from build123d import *

# Parameters (mm, degrees)
BOSS_EXTRUDE2_DEPTH           = 50
SKETCH2_R                     = 4.1
CUT_EXTRUDE1_DEPTH            = 50
SKETCH3_W                     = 12
SKETCH3_H                     = 24
CUT_EXTRUDE2_DEPTH            = 50
SKETCH4_R                     = 1.6
CUT_EXTRUDE3_DEPTH            = 50
CUT_EXTRUDE4_DEPTH            = 35
SKETCH6_R                     = 7.6
CUT_EXTRUDE5_DEPTH            = 35
CUT_EXTRUDE6_DEPTH            = 5.5
SKETCH8_R                     = 1.55
CUT_EXTRUDE7_DEPTH            = 116.876011322
CUT_EXTRUDE8_DEPTH            = 10
SKETCH10_R                    = 11
CUT_EXTRUDE9_DEPTH            = 29
SKETCH11_R                    = 1.05
SKETCH11_R_2                  = 4.75
CUT_EXTRUDE10_DEPTH           = 116.876011322
CUT_EXTRUDE11_DEPTH           = 2.5
FILLET1_R                     = 8
M3_TAPPED_HOLE3_D             = 2.5
M3_TAPPED_HOLE3_DEPTH         = 8.5
M3_TAPPED_HOLE3_CSINK_D       = 3.05
M3_TAPPED_HOLE3_CSINK_ANGLE   = 90
M3_TAPPED_HOLE3_TIP           = 0.751075774
M3_TAPPED_HOLE4_D             = 2.5
M3_TAPPED_HOLE4_DEPTH         = 7
M3_TAPPED_HOLE4_CSINK_D       = 3.05
M3_TAPPED_HOLE4_CSINK_ANGLE   = 90
M3_TAPPED_HOLE4_TIP           = 0.751075774
SKETCH15_R                    = 3.2
CUT_EXTRUDE12_DEPTH           = 1.5
CUT_EXTRUDE12_DRAFT           = -45
CUT_EXTRUDE12_PROFILE_2_DEPTH = 1.5
CUT_EXTRUDE12_PROFILE_2_DRAFT = -45
M3_TAPPED_HOLE5_D             = 2.5
M3_TAPPED_HOLE5_DEPTH         = 7
M3_TAPPED_HOLE5_CSINK_D       = 3.05
M3_TAPPED_HOLE5_CSINK_ANGLE   = 90
M3_TAPPED_HOLE5_TIP           = 0.751075774
SKETCH17_R                    = 3.2
CUT_EXTRUDE13_DEPTH           = 1.5
CUT_EXTRUDE13_DRAFT           = -45
CUT_EXTRUDE13_PROFILE_2_DEPTH = 1.5
CUT_EXTRUDE13_PROFILE_2_DRAFT = -45


with BuildPart() as part:
    # Sketch1 → Boss-Extrude2 (new body)
    with BuildSketch(Plane(origin=(0, 0, 0), x_dir=(0, 0, -1), z_dir=(1, 0, 0))):
        Polygon((0, 30), (0, 0), (-98.5, 0), (-98.5, 35), (5, 35), (5, 30), align=None)
    extrude(amount=BOSS_EXTRUDE2_DEPTH)

    # Sketch2 → Cut-Extrude1 (cut)
    with BuildSketch(Plane(origin=(50, 0, 0), x_dir=(0, 0, -1), z_dir=(1, 0, 0))):
        with Locations((-88.5, 26)):
            Circle(SKETCH2_R)
        with Locations((-8.5, 26)):
            Circle(SKETCH2_R)
    extrude(amount=-CUT_EXTRUDE1_DEPTH, mode=Mode.SUBTRACT)

    # Sketch3 → Cut-Extrude2 (cut)
    with BuildSketch(Plane(origin=(50, 0, 0), x_dir=(0, 0, -1), z_dir=(1, 0, 0))):
        with Locations((-24, 15)):
            Rectangle(SKETCH3_W, SKETCH3_H)
    extrude(amount=-CUT_EXTRUDE2_DEPTH, mode=Mode.SUBTRACT)

    # Sketch4 → Cut-Extrude3 (cut)
    with BuildSketch(Plane(origin=(50, 0, 0), x_dir=(0, 0, -1), z_dir=(1, 0, 0))):
        with Locations((-88.5, 16)):
            Circle(SKETCH4_R)
        with Locations((-68.5, 30)):
            Circle(SKETCH4_R)
        with Locations((-68.5, 5)):
            Circle(SKETCH4_R)
        with Locations((-8.5, 16)):
            Circle(SKETCH4_R)
    extrude(amount=-CUT_EXTRUDE3_DEPTH, mode=Mode.SUBTRACT)

    # Sketch5 → Cut-Extrude4 (cut)
    with BuildSketch(Plane(origin=(50, 0, 0), x_dir=(0, 0, -1), z_dir=(1, 0, 0))):
        Polygon((-65.275, 30), (-66.8875, 32.792931927), (-70.1125, 32.792931927), (-71.725, 30), (-70.1125, 27.207068073), (-66.8875, 27.207068073), align=None)
        Polygon((-85.275, 16), (-86.8875, 18.792931927), (-90.1125, 18.792931927), (-91.725, 16), (-90.1125, 13.207068073), (-86.8875, 13.207068073), align=None)
        Polygon((-65.275, 5), (-66.8875, 7.792931927), (-70.1125, 7.792931927), (-71.725, 5), (-70.1125, 2.207068073), (-66.8875, 2.207068073), align=None)
        Polygon((-5.275, 16), (-6.8875, 18.792931927), (-10.1125, 18.792931927), (-11.725, 16), (-10.1125, 13.207068073), (-6.8875, 13.207068073), align=None)
    extrude(amount=-CUT_EXTRUDE4_DEPTH, mode=Mode.SUBTRACT)

    # Sketch6 → Cut-Extrude5 (cut)
    with BuildSketch(Plane(origin=(0, 35, 0), x_dir=(1, 0, 0), z_dir=(0, 1, 0))):
        with Locations(Location((13.5, -48.5, 0), (0, 0, 270))):
            Circle(SKETCH6_R)
    extrude(amount=-CUT_EXTRUDE5_DEPTH, mode=Mode.SUBTRACT)

    # Sketch7 → Cut-Extrude6 (cut)
    with BuildSketch(Plane(origin=(0, 35, 0), x_dir=(1, 0, 0), z_dir=(0, 1, 0))):
        with BuildLine():
            Line((24.1, -36.381831822), (24.1, -60.618168178))
            ThreePointArc((24.1, -60.618168178), (13.5, -64.6), (2.9, -60.618168178))
            Line((2.9, -60.618168178), (2.9, -36.381831822))
            ThreePointArc((2.9, -36.381831822), (13.5, -32.4), (24.1, -36.381831822))
        make_face()
    extrude(amount=-CUT_EXTRUDE6_DEPTH, mode=Mode.SUBTRACT)

    # Sketch8 → Cut-Extrude7 (cut, through all)
    with BuildSketch(Plane(origin=(0, 35, 0), x_dir=(1, 0, 0), z_dir=(0, 1, 0))):
        with Locations(Location((13.5, -36.25, 0), (0, 0, 270))):
            Circle(SKETCH8_R)
        with Locations(Location((13.5, -60.75, 0), (0, 0, 270))):
            Circle(SKETCH8_R)
    extrude(amount=-CUT_EXTRUDE7_DEPTH, mode=Mode.SUBTRACT)

    # Sketch9 → Cut-Extrude8 (cut)
    with BuildSketch(Plane.XZ):
        Polygon((16.725, 60.75), (15.1125, 63.542931927), (11.8875, 63.542931927), (10.275, 60.75), (11.8875, 57.957068073), (15.1125, 57.957068073), align=None)
        Polygon((16.725, 36.25), (15.1125, 39.042931927), (11.8875, 39.042931927), (10.275, 36.25), (11.8875, 33.457068073), (15.1125, 33.457068073), align=None)
    extrude(amount=-CUT_EXTRUDE8_DEPTH, mode=Mode.SUBTRACT)

    # Sketch10 → Cut-Extrude9 (cut)
    with BuildSketch(Plane.XZ):
        with Locations(Location((36.5, 48.5, 0), (0, 0, 270))):
            Circle(SKETCH10_R)
    extrude(amount=-CUT_EXTRUDE9_DEPTH, mode=Mode.SUBTRACT)

    # Sketch11 → Cut-Extrude10 (cut, through all)
    with BuildSketch(Plane.XZ):
        with Locations(Location((30.843145751, 54.156854249, 0), (0, 0, 270))):
            Circle(SKETCH11_R)
        with Locations(Location((42.156854249, 54.156854249, 0), (0, 0, 270))):
            Circle(SKETCH11_R)
        with Locations(Location((30.843145751, 42.843145751, 0), (0, 0, 270))):
            Circle(SKETCH11_R)
        with Locations(Location((42.156854249, 42.843145751, 0), (0, 0, 270))):
            Circle(SKETCH11_R)
        with Locations(Location((36.5, 48.5, 0), (0, 0, 270))):
            Circle(SKETCH11_R_2)
    extrude(amount=-CUT_EXTRUDE10_DEPTH, mode=Mode.SUBTRACT)

    # Sketch12 → Cut-Extrude11 (cut)
    with BuildSketch(Plane(origin=(0, 35, 0), x_dir=(1, 0, 0), z_dir=(0, 1, 0))):
        Polygon((44.388142908, -42.245273756), (42.754726244, -40.611857092), (40.523437585, -41.209729086), (39.925565591, -43.441017745), (41.558982255, -45.074434409), (43.790270914, -44.476562415), align=None)
        Polygon((44.388142908, -54.754726244), (43.790270914, -52.523437585), (41.558982255, -51.925565591), (39.925565591, -53.558982255), (40.523437585, -55.790270914), (42.754726244, -56.388142908), align=None)
        Polygon((33.074434409, -43.441017745), (32.476562415, -41.209729086), (30.245273756, -40.611857092), (28.611857092, -42.245273756), (29.209729086, -44.476562415), (31.441017745, -45.074434409), align=None)
        Polygon((33.074434409, -53.558982255), (31.441017745, -51.925565591), (29.209729086, -52.523437585), (28.611857092, -54.754726244), (30.245273756, -56.388142908), (32.476562415, -55.790270914), align=None)
    extrude(amount=-CUT_EXTRUDE11_DEPTH, mode=Mode.SUBTRACT)

    # Fillet1
    fillet1_edges = [part.edges().sort_by_distance(p)[0] for p in [
        (25, 35, 98.5),
    ]]
    fillet(fillet1_edges, radius=FILLET1_R)

    # M3 Tapped Hole3
    with Locations(Plane(origin=(5, 35, 8.5), x_dir=(0, 0, 1), z_dir=(0, 1, 0))):
        with Locations((0, 0), (80, 0)):
            CounterSinkHole(M3_TAPPED_HOLE3_D / 2, M3_TAPPED_HOLE3_CSINK_D / 2, depth=M3_TAPPED_HOLE3_DEPTH, counter_sink_angle=M3_TAPPED_HOLE3_CSINK_ANGLE)
            with Locations((0, 0, -(M3_TAPPED_HOLE3_DEPTH + M3_TAPPED_HOLE3_TIP / 2))):  # 118° drill point
                Cone(0, M3_TAPPED_HOLE3_D / 2, M3_TAPPED_HOLE3_TIP, mode=Mode.SUBTRACT)

    # M3 Tapped Hole4
    with Locations(Plane(origin=(45, 35, 2.5), x_dir=(0, 0, 1), z_dir=(0, 1, 0))):
        with Locations((0, 0), (13, 0)):
            CounterSinkHole(M3_TAPPED_HOLE4_D / 2, M3_TAPPED_HOLE4_CSINK_D / 2, depth=M3_TAPPED_HOLE4_DEPTH, counter_sink_angle=M3_TAPPED_HOLE4_CSINK_ANGLE)
            with Locations((0, 0, -(M3_TAPPED_HOLE4_DEPTH + M3_TAPPED_HOLE4_TIP / 2))):  # 118° drill point
                Cone(0, M3_TAPPED_HOLE4_D / 2, M3_TAPPED_HOLE4_TIP, mode=Mode.SUBTRACT)


with BuildPart() as cut_extrude12_tool:
    # Sketch15 → Cut-Extrude12 (with draft: the straight prism first)
    with BuildSketch(Plane(origin=(0, 35, 0), x_dir=(1, 0, 0), z_dir=(0, 1, 0))):
        with Locations((45, -2.5)):
            Circle(SKETCH15_R)
    extrude(amount=-CUT_EXTRUDE12_DEPTH)
    # Cut-Extrude12: the draft: its side faces are tilted about the plane it starts from
    cut_extrude12_sides = [cut_extrude12_tool.faces().sort_by_distance(p)[0] for p in [
        (41.8, 34.25, 2.5),
    ]]
    draft(cut_extrude12_sides, Plane(origin=(0, 35, 0), x_dir=(1, 0, 0), z_dir=(0, 1, 0)), CUT_EXTRUDE12_DRAFT)


with BuildPart() as part_1:
    add(part.part)

    # Cut-Extrude12: cut by cut_extrude12_tool
    add(cut_extrude12_tool.part, mode=Mode.SUBTRACT)


with BuildPart() as cut_extrude12_profile_2_tool:
    # Sketch15 → Cut-Extrude12 profile 2 (with draft: the straight prism first)
    with BuildSketch(Plane(origin=(0, 35, 0), x_dir=(1, 0, 0), z_dir=(0, 1, 0))):
        with Locations((45, -15.5)):
            Circle(SKETCH15_R)
    extrude(amount=-CUT_EXTRUDE12_PROFILE_2_DEPTH)
    # Cut-Extrude12 profile 2: the draft: its side faces are tilted about the plane it starts from
    cut_extrude12_profile_2_sides = [cut_extrude12_profile_2_tool.faces().sort_by_distance(p)[0] for p in [
        (41.8, 34.25, 15.5),
    ]]
    draft(cut_extrude12_profile_2_sides, Plane(origin=(0, 35, 0), x_dir=(1, 0, 0), z_dir=(0, 1, 0)), CUT_EXTRUDE12_PROFILE_2_DRAFT)


with BuildPart() as part_2:
    add(part_1.part)

    # Cut-Extrude12 profile 2: cut by cut_extrude12_profile_2_tool
    add(cut_extrude12_profile_2_tool.part, mode=Mode.SUBTRACT)

    # M3 Tapped Hole5
    with Locations(Plane(origin=(5, 0, 88.5), x_dir=(0, 0, -1), z_dir=(0, -1, 0))):
        with Locations((0, 0), (13, 0)):
            CounterSinkHole(M3_TAPPED_HOLE5_D / 2, M3_TAPPED_HOLE5_CSINK_D / 2, depth=M3_TAPPED_HOLE5_DEPTH, counter_sink_angle=M3_TAPPED_HOLE5_CSINK_ANGLE)
            with Locations((0, 0, -(M3_TAPPED_HOLE5_DEPTH + M3_TAPPED_HOLE5_TIP / 2))):  # 118° drill point
                Cone(0, M3_TAPPED_HOLE5_D / 2, M3_TAPPED_HOLE5_TIP, mode=Mode.SUBTRACT)


with BuildPart() as cut_extrude13_tool:
    # Sketch17 → Cut-Extrude13 (with draft: the straight prism first)
    with BuildSketch(Plane.XZ):
        with Locations((5, 88.5)):
            Circle(SKETCH17_R)
    extrude(amount=-CUT_EXTRUDE13_DEPTH)
    # Cut-Extrude13: the draft: its side faces are tilted about the plane it starts from
    cut_extrude13_sides = [cut_extrude13_tool.faces().sort_by_distance(p)[0] for p in [
        (1.8, 0.75, 88.5),
    ]]
    draft(cut_extrude13_sides, Plane.XZ, CUT_EXTRUDE13_DRAFT)


with BuildPart() as part_3:
    add(part_2.part)

    # Cut-Extrude13: cut by cut_extrude13_tool
    add(cut_extrude13_tool.part, mode=Mode.SUBTRACT)


with BuildPart() as cut_extrude13_profile_2_tool:
    # Sketch17 → Cut-Extrude13 profile 2 (with draft: the straight prism first)
    with BuildSketch(Plane.XZ):
        with Locations((5, 75.5)):
            Circle(SKETCH17_R)
    extrude(amount=-CUT_EXTRUDE13_PROFILE_2_DEPTH)
    # Cut-Extrude13 profile 2: the draft: its side faces are tilted about the plane it starts from
    cut_extrude13_profile_2_sides = [cut_extrude13_profile_2_tool.faces().sort_by_distance(p)[0] for p in [
        (1.8, 0.75, 75.5),
    ]]
    draft(cut_extrude13_profile_2_sides, Plane.XZ, CUT_EXTRUDE13_PROFILE_2_DRAFT)


with BuildPart() as part_4:
    add(part_3.part)

    # Cut-Extrude13 profile 2: cut by cut_extrude13_profile_2_tool
    add(cut_extrude13_profile_2_tool.part, mode=Mode.SUBTRACT)


solid = part_4.part
Model file for the job. Use its own axes, mm. A direction names the side the tool comes from. Coordinates: 2 decimals unless noted, no trailing zeros. Order: outer loops, then holes, each group sorted by start corner. A loop starts at its lowest first (then second) coordinate and runs counter-clockwise, first axis right, second up. Notation, with made-up numbers: (-9, -18.75) -> (34, -18.75) arc R17 ccw to (34, -0.75) -> close; hole circle Ø2 at (-23, 38.5). An arc over 180 degrees is marked (long way). Return JSON: item names as keys, results as strings. Group by question number.
Item 1: Saw through at A-A on y = 26. Write the cut outline in (x, z).
Item 2: Saw through at C-C on x = 13.5. State how many separate pieces and enclosed holes the cut face has, then the cut area to 3 significant figures.
Item 3: Saw through at B-B on z = 68.5. Write the cut outline in (x, y).
Item 4: Tool access for faces 4 (the flat face through (15, 17, 7)), 5 (the flat face through (25, 3, 24)), 6 (the cylindrical face through (4.521, 4.288, 89.655)), 7 (the flat face through (30.34, 33.77, 52.22)), 8 (the flat face through (50, 18, 46)): list every direction of +Z, -Z, +X, -X, +Y, -Y with a clear straight run to the whole face (end or side of a thin tool).
Item 5: Flat gauge pins, fed straight in: P1, Ø1.3, axis at x = 42.5, z = 53.5, coming from the +Y side; P2, Ø1, axis at x = 38, y = 16.5, coming from the -Z side; P3, Ø5.5, axis at x = 30.5, z = -3, coming from the -Y side. Where does each tip first touch, or does it go through?
Item 6: Wall check: line 1 along X through (y, z) = (32.2, 48.5); line 2 along Z through (x, y) = (39, 12.5); line 3 along Z through (x, y) = (20.5, 32.5). Give the ranges that are in metal, low to high. Write a range as [from, to].
Item 7: Pull direction Y, two halves, no side cores. Call faces 1 (the flat face through (32.745, 17.416, 10.907)), 2 (the flat face through (2.9, 32, 49)), 3 (the flat face through (25, 30, -3)): pulls with the +Y half, pulls with the -Y half, needs draft (parallel to the pull), parting line crosses it, or undercut.
Values found:
{
 "1": {"outline": "(0, 0) -> (50, 0) -> (50, 4.4) -> (0, 4.4) -> close; (0, 12.6) -> (50, 12.6) -> (50, 18) -> (0, 18) -> close; (0, 30) -> (50, 30) -> (50, 84.4) -> (0, 84.4) -> close; (0, 92.6) -> (50, 92.6) -> (50, 98.5) -> (0, 98.5) -> close; hole circle Ø15.2 at (13.5, 48.5); hole circle Ø3.1 at (13.5, 36.25); hole circle Ø3.1 at (13.5, 60.75); hole circle Ø22 at (36.5, 48.5)"},
 "2": {"separate pieces": "4", "enclosed holes": "7", "area": "2,170 mm2"},
 "3": {"outline": "(0, 0) -> (50, 0) -> (50, 2.21) -> (15, 2.21) -> (15, 3.4) -> (0, 3.4) -> close; (0, 6.6) -> (15, 6.6) -> (15, 7.79) -> (50, 7.79) -> (50, 27.21) -> (15, 27.21) -> (15, 28.4) -> (0, 28.4) -> close; (0, 31.6) -> (15, 31.6) -> (15, 32.79) -> (50, 32.79) -> (50, 35) -> (0, 35) -> close"},
 "4": {"face 4": "+X", "face 5": "+X, -X", "face 6": "-Y", "face 7": "+Y", "face 8": "+Z, -Z, +X, +Y, -Y"},
 "5": {"P1": "stops at y = 32.5", "P2": "stops at z = 0", "P3": "stops at y = 30"},
 "6": {"line 1": "x = [0, 2.9], [24.1, 31.75], [41.25, 50]", "line 2": "z = [0, 18], [30, 37.79], [59.21, 98.5]", "line 3": "z = [-5, 34], [63, 66.72], [70.28, 96.31]"},
 "7": {"face 1": "undercut", "face 2": "needs draft", "face 3": "pulls with the -Y half"}
}
